For this review, take the finished solid that the model builds, in its own axes (mm). A direction names the side the tool comes from. Round coordinates to 2 decimals unless told otherwise and drop trailing zeros. Order: outer loops, then holes, each group sorted by start corner. A loop starts at its lowest first (then second) coordinate and runs counter-clockwise, first axis right, second up. Notation, with made-up numbers: (-39.5, 47.5) -> (-1.5, 47.5) arc R20 ccw to (-1.5, 71.5) -> close; hole circle Ø1 at (31, 29). An arc over 180 degrees is marked (long way). Put each result on its own line as item: value. Start each with the question number.
```python
from build123d import *

# Parameters (mm, degrees)
CHAMFER1_SIZE = 0.5


with BuildPart() as part:
    # Sketch1 → Revolve1 (revolve)
    with BuildSketch(Plane(origin=(0, 0, 0), x_dir=(0, 0, -1), z_dir=(1, 0, 0))):
        Polygon((0, 0), (35, 0), (38, 3), (50, 3), (50, 9), (0, 9), align=None)
    revolve(axis=Axis((0, 0, 494.673459935), (0, 0, -1)))

    # Chamfer1
    chamfer1_edges = [part.edges().sort_by_distance(p)[0] for p in [
        (0, -9, 0),
        (0, -9, -50),
        (0, -3, -50),
    ]]
    chamfer(chamfer1_edges, length=CHAMFER1_SIZE)


solid = part.part
```
Item 1: Consider section B-B, the plane z = -25.5. Write out the cut boundary in (x, y), plus the area to 3 significant figures.
Item 2: Insertion check: pin 1 Ø2 at (x, z) = (4, -32) entering from +Y; pin 2 Ø8 at (y, z) = (6, -40.5) entering from -X; pin 3 Ø8 at (x, z) = (-7, -38.5) entering from -Y. Each pin has a flat end and moves straight along its axis. Give the tip position at first contact, or say it passes through.
Item 3: Consider section A-A, the plane z = -40.5. Write out the cut boundary in (x, y).
Item 4: Mouldability with a two-part tool opening along X and no side actions: class faces 3 (the face through (0, 0, 0)), 4 (the face through (8.923, -1.172, -24.657)), 5 (the face through (-1, 0, -36)) as +X half, -X half, draft (parallel to the pull), parting line (faces both ways), or undercut.
Item 5: Tool access review of faces 1 (the face through (0, -4, -50)), 2 (the face through (0, -3, -44)): name each direction out of +Z, -Z, +X, -X, +Y, -Y from which nothing blocks a thin tool from reaching the whole face with its end or side.
Item 6: For L1, parallel to X at y = 0, z = -40.25; L2, parallel to Y at x = 1.25, z = -28; L3, parallel to X at y = 1, z = -27, list the stretches that pass through material, from the lowest coordinate up.
Evaluation:
1. outline: circle Ø18 at (0, 0)
1. area: 254 mm^2
2. pin 1: stops at y = 8.49
2. pin 2: stops at x = -8.77
2. pin 3: stops at y = -8.49
3. outline: circle Ø18 at (0, 0); hole circle Ø6 at (0, 0)
4. face 3: draft
4. face 4: parting line
4. face 5: undercut
5. face 1: -Z, +X, -X, +Y, -Y
5. face 2: -Z
6. L1: x = -9 to -3, 3 to 9
6. L2: y = -8.91 to 8.91
6. L3: x = -8.94 to 8.94
